Here's how the part is built. I have some questions about the finished solid (model axes, mm). Face numbers are marked on the shaded views. Give positions to 0.01 mm unless a question says otherwise; leave off trailing zeros. Write each loop counter-clockwise with the first axis right and the second up, starting at its lowest first coordinate (ties: lowest second). Pieces come first, ordered by that corner, then holes. Notation, with made-up numbers: (48.5, -11) - (61.5, -11) arc R14 cw to (61.5, 5) - close; hole circle Ø6 at (66.25, 74.5). An arc over 180 degrees is marked (long way). One line per item, written item: value. Start each with the question number.
1) Imagine slicing it at B-B on z = 0. Write out the boundary of the cut face in (x, y).
2) Imagine slicing it at A-A on x = 0. Write out the boundary of the cut face in (y, z).
3) Imagine slicing it at C-C on y = 8.5. Write out the boundary of the cut face in (x, z), plus the area to 3 significant figures.
4) Imagine slicing it at D-D on x = -11. Write out the boundary of the cut face in (y, z), plus the area to 3 significant figures.
5) We'd pull the mould along Z, two halves only. Please class the marked faces 1, 2 and 3: +Z half, -Z half, draft (parallel to the pull), parting line (faces both ways), or undercut.
6) I'm going to push flat-ended pins straight in: P1, Ø5, axis at y = 9, z = -6, coming from the +X side; P2, Ø4.5, axis at x = 24, z = 0, coming from the +Y side; P3, Ø3, axis at y = 3.5, z = 12, coming from the +X side. Where does each tip first touch, or does it pass through?
7) Please list where these lines run through material, in increasing order: L1, parallel to X at y = 0.8, z = 0; L2, parallel to X at y = 11, z = 0; L3, parallel to Y at x = -5.5, z = -19.5. Write a range as [from, to].
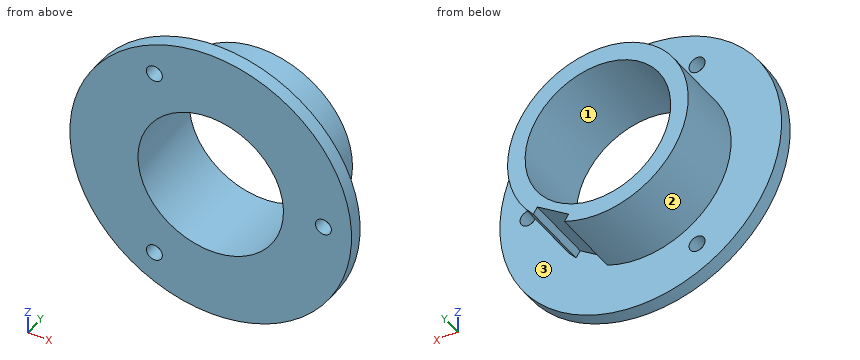
from build123d import *

# Parameters (mm, degrees)
SKETCH2_R          = 30
SKETCH2_R_2        = 19.25
FLANG_DEPTH        = 3
SKETCH2_3_R        = 19.25
SKETCH2_3_R_2      = 15.5
SKIRT_DEPTH        = 18
SKETCH3_R          = 1.7
HOLES_BOLTS_DEPTH  = 46
SERVICE_SLOT_DEPTH = 46


with BuildPart() as part:
    # Sketch2 → flang (new body)
    with BuildSketch(Plane(origin=(0, 0, 0), x_dir=(1, 0, 0), z_dir=(0, 1, 0))):
        with Locations(Location((0, 0, 0), (0, 0, 270))):
            Circle(SKETCH2_R)
        with Locations(Location((0, 0, 0), (0, 0, 270))):
            Circle(SKETCH2_R_2, mode=Mode.SUBTRACT)
    extrude(amount=FLANG_DEPTH)

    # Sketch2_3 → skirt (add)
    with BuildSketch(Plane(origin=(0, 0, 0), x_dir=(1, 0, 0), z_dir=(0, 1, 0))):
        with Locations(Location((0, 0, 0), (0, 0, 270))):
            Circle(SKETCH2_3_R)
        with Locations(Location((0, 0, 0), (0, 0, 270))):
            Circle(SKETCH2_3_R_2, mode=Mode.SUBTRACT)
    extrude(amount=SKIRT_DEPTH)

    # Sketch3 → holes_bolts (cut, through all)
    with BuildSketch(Plane(origin=(0, 3, 0), x_dir=(1, 0, 0), z_dir=(0, 1, 0))):
        with Locations(Location((24, 0, 0), (0, 0, 270))):
            Circle(SKETCH3_R)
        with Locations(Location((-12, -20.784609691, 0), (0, 0, 270))):
            Circle(SKETCH3_R)
        with Locations(Location((-12, 20.784609691, 0), (0, 0, 270))):
            Circle(SKETCH3_R)
    extrude(amount=-HOLES_BOLTS_DEPTH, mode=Mode.SUBTRACT)

    # Sketch8 → service_slot (cut, through all)
    with BuildSketch(Plane(origin=(0, 3, 0), x_dir=(1, 0, 0), z_dir=(0, 1, 0))):
        Polygon((14.000367572, 13.804064903), (7.342096898, 18.238862715), (6.233397445, 16.574295047), (12.891668119, 12.139497235), align=None)
    extrude(amount=SERVICE_SLOT_DEPTH, mode=Mode.SUBTRACT)


solid = part.part
Numbers:
1. outline: (-30, 0) - (-15.5, 0) - (-15.5, 18) - (-19.25, 18) - (-19.25, 3) - (-30, 3) - close; (15.5, 0) - (22.3, 0) - (22.3, 3) - (19.25, 3) - (19.25, 18) - (15.5, 18) - close; (25.7, 0) - (30, 0) - (30, 3) - (25.7, 3) - close
2. outline: (0, -30) - (3, -30) - (3, -19.25) - (18, -19.25) - (18, -15.5) - (0, -15.5) - close; (0, 15.5) - (18, 15.5) - (18, 19.25) - (3, 19.25) - (3, 30) - (0, 30) - close
3. outline: (6.23, -16.57) - (12.89, -12.14) - (13.77, -13.45) arc R19.25 ccw (long way) to (7.11, -17.89) - close; hole circle Ø31 at (0, 0)
3. area: 395 mm^2
4. outline: (0, -27.91) - (3, -27.91) - (3, -22.16) - (0, -22.16) - close; (0, -19.41) - (3, -19.41) - (3, -15.8) - (18, -15.8) - (18, -10.92) - (0, -10.92) - close; (0, 10.92) - (18, 10.92) - (18, 15.8) - (3, 15.8) - (3, 19.41) - (0, 19.41) - close; (0, 22.16) - (3, 22.16) - (3, 27.91) - (0, 27.91) - close
4. area: 232 mm^2
5. face 1: undercut
5. face 2: parting line
5. face 3: draft
6. P1: x = 18.93
6. P2: y = 3
6. P3: x = 28.07
7. L1: [-30, -15.5], [15.5, 22.3], [25.7, 30]
7. L2: [-19.25, -15.5], [15.5, 19.25]
7. L3: [0, 3]
